from build123d import *


# Not quite as in the source:
# - a pattern or mirror of a feature is missing from the dataset's text; its kind, count and spacing are read off the source's solid


with BuildPart() as f1:
    # F0 (on Front) → F1 (revolve)
    with BuildSketch(Plane.XZ):
        with BuildLine():
            Line((27.2213151776, 10), (17.2213151776, 10))
            ThreePointArc((17.2213151776, 10), (19.9141581908, 0), (17.2213151776, -10))
            Line((17.2213151776, -10), (27.2213151776, -10))
            Line((27.2213151776, -10), (27.2213151776, 10))
        make_face()
        with BuildLine():
            ThreePointArc((27.2213151776, -10), (29, 0), (27.2213151776, 10))
            Line((27.2213151776, 10), (27.2213151776, -10))
        make_face()
    revolve(axis=Axis((0, 0, -0.0082536135), (0, 0, -1)))

    # F2 (on Top) → F3 (revolve, cut)
    with BuildSketch(Plane.XY):
        Polygon((0, 30.5), (0, 21.5), (9, 30.5), align=None)
    f3 = revolve(axis=Axis((0, 26, 0), (0, -1, 0)), mode=Mode.SUBTRACT)

    # F3_copies: F3 across plane
    add(f3.mirror(Plane(origin=(0, 0, 0), x_dir=(0, 0, -1), z_dir=(0, -1, 0))), mode=Mode.SUBTRACT)

    # F4 (on Top) → F5 (revolve)
    with BuildSketch(Plane.XY):
        Polygon((-10.5096189432, 0), (-23.5, 7.5), (-23.5, 0), align=None)
    f5 = revolve(axis=Axis((-17.0048094716, 0, 0), (-1, 0, 0)))

    # F5_copies: F5 across plane
    add(f5.mirror(Plane(origin=(0, 0, 0), x_dir=(0, 0, 1), z_dir=(1, 0, 0))))


solid = f1.part
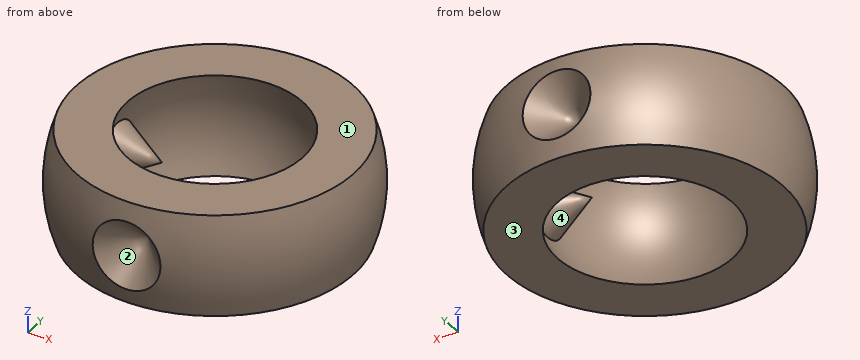
The model under review builds one solid part; all positions refer to its coordinate system, in mm. Face numbers are marked on the shaded views. A direction names the side the tool comes from. Give positions to 0.01 mm unless a question says otherwise; leave off trailing zeros. Order: outer loops, then holes, each group sorted by start corner. A loop starts at its lowest first (then second) coordinate and runs counter-clockwise, first axis right, second up. Notation, with made-up numbers: (-19, 64.5) -> (10, 64.5) arc R33 cw to (10, 92.5) -> close; hole circle Ø7 at (-18.75, 38). An arc over 180 degrees is marked (long way). Write item = value, one per line. Start each with the question number.
(1) For L1, parallel to Y at x = -15, z = -1.5; L2, parallel to Y at x = 10, z = -0.5; L3, parallel to Y at x = -9, z = 5.5, list the stretches that pass through material, from the lowest coordinate up. Write a range as from..to.
(2) Take a section at B-B (y = 15). Write out the cut boundary in (x, z).
(3) Take a section at D-D (z = -8). Write out the cut boundary in (x, y).
(4) Take a section at C-C (x = -24). Write out the cut boundary in (y, z), plus the area to 3 significant figures.
(5) Take a section at A-A (y = -8). Write out the cut boundary in (x, z), plus the area to 3 significant figures.
(6) Draft analysis for pull direction X (two halves, no side actions). For the marked faces 1 and 2, state which applies: +X half, -X half, draft (parallel to the pull), parting line (faces both ways), or undercut.
(7) Tool access review of the marked faces 3 and 4: name each direction out of +Z, -Z, +X, -X, +Y, -Y from which nothing blocks a thin tool from reaching the whole face with its end or side.
(8) For pin 1 Ø3 at (x, z) = (23, -4.5) entering from +Y; pin 2 Ø2 at (y, z) = (11, 2) entering from +X; pin 3 Ø3 at (x, z) = (18.5, 7) entering from +Y, all flat-tipped, find the tip position at first contact; note any pin that passes through.
Returned:
q1.L1 = -24.77..-13.01, -2.11..2.11, 13.01..24.77
q1.L2 = -27.22..-17.21, 17.21..27.22
q1.L3 = -27.01..-16.89, 16.89..27.01
q2.outline = (-22.72, -10) -> (-8.46, -10) arc R13.1 cw to (-8.46, 10) -> (-22.72, 10) arc R24.82 ccw to start; (8.46, -10) -> (22.72, -10) arc R24.82 ccw to (22.72, 10) -> (8.46, 10) arc R13.1 cw to start
q3.outline = circle Ø55.75 at (0, 0); hole circle Ø36.47 at (0, 0)
q4.outline = (-12.85, -10) -> (12.85, -10) arc R16.28 ccw to (12.85, 10) -> (-12.85, 10) arc R16.28 ccw to start
q4.area = 607 mm²
q5.outline = (-26.02, -10) -> (-15.25, -10) arc R18.24 cw to (-15.25, 10) -> (-26.02, 10) arc R27.87 ccw to start; (15.25, -10) -> (26.02, -10) arc R27.87 ccw to (26.02, 10) -> (15.25, 10) arc R18.24 cw to start
q5.area = 400 mm²
q6.face_1 = draft
q6.face_2 = undercut
q7.face_3 = -Z, +X, -X, +Y, -Y
q7.face_4 = none
q8.pin_1 = 18.97
q8.pin_2 = 27.15
q8.pin_3 = 22.51
